from build123d import *

# Parameters (mm, degrees)
F0_W     = 936.625
F0_H     = 457.2
F1_DEPTH = 254
F2_W     = 898.525
F2_H     = 419.1
F3_DEPTH = 234.95
F4_W     = 958.85
F4_H     = 327.025
F5_DEPTH = 19.05


with BuildPart() as f1:
    # F0 (on Top) → F1 (new body)
    with BuildSketch(Plane.XY):
        with Locations((-12.105351, 5.909053)):
            Rectangle(F0_W, F0_H)
    extrude(amount=F1_DEPTH)

    # F2 (on face) → F3 (cut)
    with BuildSketch(Plane.XY.offset(254)):
        with Locations((-12.105351, 5.909053)):
            Rectangle(F2_W, F2_H)
    extrude(amount=-F3_DEPTH, mode=Mode.SUBTRACT)

    # F4 (on face) → F5 (join)
    with BuildSketch(Plane.XZ.offset(222.690947)):
        with Locations((-12.105351, 138.1125)):
            Rectangle(F4_W, F4_H)
    extrude(amount=F5_DEPTH)


solid = f1.part
Geometry check sheet. Reference: the model listing, model coordinates, mm. A direction names the side the tool comes from. Give positions to 0.01 mm unless a question says otherwise; leave off trailing zeros. Loops run counter-clockwise (first coordinate to the right, second up) from the corner with the lowest first, then second, coordinate; pieces in that order, holes last. Notation, with made-up numbers: M -38.5,-39.5 L 9.5,-39.5 A11 ccw 9.5,-22.5 Z; hole C -22.75,45.25 d10. An arc over 180 degrees is marked long. Answer as a JSON object with one key per item and string values. Group by question number.
Item 1: Sectioned sample at B-B on y = 151. Record the boundary of the cut face in (x, z), plus the area to 3 significant figures.
Item 2: Access from +Z, -Z, +X, -X, +Y, -Y to the whole of each face (thin tool, end or side, straight path). Record for faces 5 (the flat face through (-19, 9, 0)), 6 (the flat face through (467.32, -232, 136)), 7 (the flat face through (-18, 9, 19.05)).
Item 3: Mould release check, pull along X, two halves, no side actions. Record for faces 1 (the flat face through (-153, 227, 254)), 2 (the flat face through (456.207, 3, 125)), 3 (the flat face through (-461.368, 3, 138)), 4 (the flat face through (-480.418, 3, 125)): pulls with the +X half, pulls with the -X half, needs draft (parallel to the pull), parting line crosses it, or undercut.
Item 4: Material ranges on L1, parallel to X at y = 42, z = 136; L2, parallel to Y at x = 413, z = 144; L3, parallel to Z at x = 387, y = 117.5, recorded low to high.
Item 5: Gauge pin test, flat ends, axial feed: pin 1 (1 mm diameter, centred on x = 346, y = -99.5, fed in from +Z); pin 2 (12 mm diameter, centred on y = 41, z = 124, fed in from +X); pin 3 (1.5 mm diameter, centred on x = 314, y = -33, fed in from -Z). Record the tip position at first contact, or that the pin passes through.
Item 6: Sectioned sample at A-A on z = 165.5. Record the boundary of the cut face in (x, y).
Item 7: Sectioned sample at C-C on x = -323.5. Record the boundary of the cut face in (y, z) (3 decimals).
Findings below:
{
 "1": {"outline": "M -480.42,0 L 456.21,0 L 456.21,254 L 437.16,254 L 437.16,19.05 L -461.37,19.05 L -461.37,254 L -480.42,254 Z", "area": "26,800 mm2"},
 "2": {"face 5": "-Z, +X, -X, +Y", "face 6": "+Z, -Z, +X, +Y, -Y", "face 7": "+Z"},
 "3": {"face 1": "needs draft", "face 2": "pulls with the +X half", "face 3": "undercut", "face 4": "pulls with the -X half"},
 "4": {"L1": "-480.42 to -461.37, 437.16 to 456.21", "L2": "-241.74 to -203.64, 215.46 to 234.51", "L3": "0 to 19.05"},
 "5": {"pin 1": "z = 19.05", "pin 2": "x = 456.21", "pin 3": "z = 0"},
 "6": {"outline": "M -491.53,-241.74 L 467.32,-241.74 L 467.32,-222.69 L 456.21,-222.69 L 456.21,234.51 L -480.42,234.51 L -480.42,-222.69 L -491.53,-222.69 Z; hole M -461.37,-203.64 L 437.16,-203.64 L 437.16,215.46 L -461.37,215.46 Z"},
 "7": {"outline": "M -241.741,-25.4 L -222.691,-25.4 L -222.691,0 L 234.509,0 L 234.509,254 L 215.459,254 L 215.459,19.05 L -203.641,19.05 L -203.641,254 L -222.691,254 L -222.691,301.625 L -241.741,301.625 Z"}
}
